from build123d import *

# Parameters (mm, degrees)
SKETCH1_W           = 1343.502884254
SKETCH1_H           = 1343.502884254
SKETCH1_R           = 5
SKETCH1_W_2         = 1281.27748751
SKETCH1_H_2         = 1281.27748751
BOSS_EXTRUDE1_DEPTH = 10


with BuildPart() as part:
    # Sketch1 → Boss-Extrude1 (new body)
    with BuildSketch(Plane.XY):
        Rectangle(SKETCH1_W, SKETCH1_H)
        with Locations((-656.195092941, 656.195092941)):
            Circle(SKETCH1_R, mode=Mode.SUBTRACT)
        with Locations((656.195092941, 656.195092941)):
            Circle(SKETCH1_R, mode=Mode.SUBTRACT)
        with Locations((656.195092941, -656.195092941)):
            Circle(SKETCH1_R, mode=Mode.SUBTRACT)
        with Locations((-656.195092941, -656.195092941)):
            Circle(SKETCH1_R, mode=Mode.SUBTRACT)
        Rectangle(SKETCH1_W_2, SKETCH1_H_2, mode=Mode.SUBTRACT)
    extrude(amount=BOSS_EXTRUDE1_DEPTH)


solid = part.part
Source: CAD feature listing. Evaluate the final solid. Frame: model axes, mm. Round coordinates to 2 decimals unless told otherwise and drop trailing zeros. Loops run counter-clockwise (first coordinate to the right, second up) from the corner with the lowest first, then second, coordinate; pieces in that order, holes last.
Q1. Mould query, pull axis Z, two halves, no side actions, for faces 1 (the face through (-53, -644, 10)), 2 (the face through (-53, -644, 0)). Classes: pulls with the +Z half, pulls with the -Z half, needs draft (parallel to the pull), parting line crosses it, or undercut.
Q2. Ray query, line 1 (X direction, y = 572.5, z = 8.25). Return the intervals inside material, ascending.
Q3. Section C-C, the plane z = 6. Return loops of the section in (x, y), plus the area to 3 significant figures.
Q4. Section A-A, the plane y = 140.5. Return loops of the section in (x, z), plus the area to 3 significant figures.
Solutions:
1. face 1: pulls with the +Z half
1. face 2: pulls with the -Z half
2. line 1: x = -671.75 to -640.64, 640.64 to 671.75
3. outline: (-671.75, -671.75) - (671.75, -671.75) - (671.75, 671.75) - (-671.75, 671.75) - close; hole circle Ø10 at (-656.2, -656.2); hole circle Ø10 at (-656.2, 656.2); hole (-640.64, -640.64) - (640.64, -640.64) - (640.64, 640.64) - (-640.64, 640.64) - close; hole circle Ø10 at (656.2, -656.2); hole circle Ø10 at (656.2, 656.2)
3. area: 163,000 mm2
4. outline: (-671.75, 0) - (-640.64, 0) - (-640.64, 10) - (-671.75, 10) - close; (640.64, 0) - (671.75, 0) - (671.75, 10) - (640.64, 10) - close
4. area: 622 mm2
